```python
from build123d import *

# Parameters (mm, degrees)
STOCK_WING_STRUCTURESIZING_1_START = 350.5
STOCK_WING_STRUCTURESIZING_1_DEPTH = 3
CUT_EXTRUDE2_DEPTH                 = 278.894871602
CUT_EXTRUDE2_DEPTH_BACK            = 278.894871602
SKETCH3_R                          = 8
SKETCH3_W                          = 3
SKETCH3_H                          = 18.234468085
CUT_EXTRUDE5_DEPTH                 = 278.894871602
CUT_EXTRUDE5_DEPTH_BACK            = 278.894871602
SKETCH6_W                          = 72
SKETCH6_H                          = 36.832163157
SKETCH7_W                          = 3
SKETCH7_H                          = 29.829109924
CUT_EXTRUDE6_DEPTH                 = 3
BOSS_EXTRUDE1_DEPTH                = 3
SKETCH9_R                          = 7.192226029
SKETCH9_R_2                        = 11.636406179
SKETCH9_R_3                        = 13.307061318
SKETCH9_R_4                        = 12.161876466
SKETCH9_R_5                        = 9.990979792
SKETCH9_R_6                        = 6.753270012
CUT_EXTRUDE7_DEPTH                 = 10


# Read off the part's stored shape, not the designer's step: Stock-Wing_structureSizing-1
with BuildPart() as part:
    # Stock-Wing_structureSizing-1 outline → Stock-Wing_structureSizing-1 (new body)
    with BuildSketch(Plane.XY.offset(STOCK_WING_STRUCTURESIZING_1_START)):
        with BuildLine():
            Line((276.744987748, -9.975467242), (276.744987748, -2.791972149))
            add(Edge.make_bspline(
                [(276.744987748, -2.791972149), (265.3857023, -0.102525952), (253.985388892, 2.407220527), (231.123115134, 7.137179769), (219.66894224, 9.35664169), (202.450532833, 12.449607831), (196.704666185, 13.440005467), (185.197495984, 15.322846112), (179.436018194, 16.214183509), (167.896810084, 17.893728146), (162.119320772, 18.683464695), (150.549559093, 20.169132171), (144.757676972, 20.867539393), (133.154760401, 22.142823058), (127.340720117, 22.719276226), (115.726117513, 23.709424358), (109.921864102, 24.123286294), (92.520744809, 25.054695045), (80.935765142, 25.255529424), (63.589579679, 24.723206588), (57.812696472, 24.40777964), (49.15741104, 23.667136334), (46.27396258, 23.376378774), (40.511150261, 22.68602794), (37.631848569, 22.284778258), (31.878918329, 21.331115885), (29.005409213, 20.775520933), (24.699904445, 19.815325722), (23.265457389, 19.476044022), (20.398415094, 18.74813831), (18.963740816, 18.357002163), (16.106748162, 17.497000764), (14.692710081, 17.03099603), (11.902486035, 16.004726933), (10.526189891, 15.444736939), (8.50012674, 14.509175123), (7.830361802, 14.183402304), (6.512563898, 13.477739544), (5.865248411, 13.093583044), (4.633392785, 12.255605476), (4.045066641, 11.801499914), (3.209118512, 11.061128735), (2.938431583, 10.804207958), (2.416562808, 10.265550671), (2.165207772, 9.983507914), (1.696102707, 9.397220013), (1.477442994, 9.09171798), (1.085439515, 8.447078561), (0.915512906, 8.113897404), (0.714798114, 7.59155933), (0.657190766, 7.413573783), (0.566275814, 7.047480769), (0.533643429, 6.859526942), (0.498702003, 6.485823786), (0.495732967, 6.298500114), (0.52230969, 5.922794269), (0.553180601, 5.733657444), (0.641956646, 5.367254731), (0.699629973, 5.188174612), (0.835770495, 4.836464845), (0.914681224, 4.663114785), (1.173802922, 4.160517642), (1.376431151, 3.845824341), (1.822835658, 3.244491079), (2.068245893, 2.956719217), (2.585349641, 2.410512622), (2.856205808, 2.152934366), (3.699269455, 1.418677094), (4.302923323, 0.981675809), (5.262649419, 0.394618321), (5.591648375, 0.21018796), (6.254696782, -0.135942129), (6.589931521, -0.298692503), (7.602521133, -0.767803382), (8.28593821, -1.057311971), (9.662885491, -1.60821635), (10.357226689, -1.867357708), (12.455074514, -2.603572901), (13.873250521, -3.039868309), (16.739197416, -3.830190303), (18.188973825, -4.184254143), (22.54237297, -5.143962802), (25.459339583, -5.655261329), (31.306270814, -6.564233952), (34.235701619, -6.966574468), (40.104165427, -7.687316125), (43.043386977, -8.004069053), (51.874086741, -8.840379009), (57.778366073, -9.248032718), (66.64804678, -9.743583642), (69.60756187, -9.887823594), (75.525585547, -10.141245843), (78.484610817, -10.250077692), (84.402679828, -10.443151081), (87.361723417, -10.527595381), (93.279819329, -10.684856962), (96.238871496, -10.7578835), (111.034153794, -11.094438823), (122.870449548, -11.270610432), (140.625005024, -11.385979432), (146.54320834, -11.400264082), (158.379650661, -11.381324799), (164.297889136, -11.348805922), (176.134384089, -11.259801078), (182.052639742, -11.204415721), (193.889154401, -11.089178887), (199.807414258, -11.02819544), (217.562198328, -10.839257795), (229.398721047, -10.713290888), (253.0718283, -10.379069852), (264.908412973, -10.164021277), (276.744987748, -9.975467242)],
                knots=[0, 0, 0, 0, 0.0625, 0.0625, 0.125, 0.125, 0.15625, 0.15625, 0.1875, 0.1875, 0.21875, 0.21875, 0.25, 0.25, 0.28125, 0.28125, 0.3125, 0.3125, 0.375, 0.375, 0.40625, 0.40625, 0.421875, 0.421875, 0.4375, 0.4375, 0.453125, 0.453125, 0.4609375, 0.4609375, 0.46875, 0.46875, 0.4765625, 0.4765625, 0.484375, 0.484375, 0.48828125, 0.48828125, 0.4921875, 0.4921875, 0.49609375, 0.49609375, 0.498046875, 0.498046875, 0.5, 0.5, 0.501953125, 0.501953125, 0.50390625, 0.50390625, 0.504882813, 0.504882813, 0.505859375, 0.505859375, 0.506835938, 0.506835938, 0.5078125, 0.5078125, 0.508789063, 0.508789063, 0.509765625, 0.509765625, 0.51171875, 0.51171875, 0.513671875, 0.513671875, 0.515625, 0.515625, 0.51953125, 0.51953125, 0.521484375, 0.521484375, 0.5234375, 0.5234375, 0.52734375, 0.52734375, 0.53125, 0.53125, 0.5390625, 0.5390625, 0.546875, 0.546875, 0.5625, 0.5625, 0.578125, 0.578125, 0.59375, 0.59375, 0.625, 0.625, 0.640625, 0.640625, 0.65625, 0.65625, 0.671875, 0.671875, 0.6875, 0.6875, 0.75, 0.75, 0.78125, 0.78125, 0.8125, 0.8125, 0.84375, 0.84375, 0.875, 0.875, 0.9375, 0.9375, 1, 1, 1, 1], degree=3))
        make_face()
    extrude(amount=STOCK_WING_STRUCTURESIZING_1_DEPTH)

    # Sketch3 → Cut-Extrude2 (cut, two sides: drawn at the far end of the back side and taken through both)
    with BuildSketch(Plane.XY.offset(353.5).offset(-CUT_EXTRUDE2_DEPTH_BACK)):
        with Locations((76.810751166, 3.840845639)):
            Circle(SKETCH3_R)
        with Locations((62.810751166, 15.958079682)):
            Rectangle(SKETCH3_W, SKETCH3_H)
        with Locations((90.810751166, 15.958079682)):
            Rectangle(SKETCH3_W, SKETCH3_H)
    extrude(amount=CUT_EXTRUDE2_DEPTH + CUT_EXTRUDE2_DEPTH_BACK, mode=Mode.SUBTRACT)

    # Sketch6 → Cut-Extrude5 (cut, two sides: drawn at the far end of the back side and taken through both)
    with BuildSketch(Plane.XY.offset(353.5).offset(-CUT_EXTRUDE5_DEPTH_BACK)):
        with Locations((240.744987748, -6.383719695)):
            Rectangle(SKETCH6_W, SKETCH6_H)
    extrude(amount=CUT_EXTRUDE5_DEPTH + CUT_EXTRUDE5_DEPTH_BACK, mode=Mode.SUBTRACT)

    # Sketch7 → Cut-Extrude6 (cut)
    with BuildSketch(Plane.XY.offset(353.5)):
        with Locations((1.5, 14.914554962)):
            Rectangle(SKETCH7_W, SKETCH7_H)
    extrude(amount=-CUT_EXTRUDE6_DEPTH, mode=Mode.SUBTRACT)

    # Sketch8 → Boss-Extrude1 (add)
    with BuildSketch(Plane.XY.offset(353.5)):
        Polygon((14.079741692, 16.8), (3, 16.8), (3, 10.856999155), (0, 10.856999155), (0, 2.029447684), (3, 2.029447684), (3, 0), (5.994622402, 0), align=None)
        Polygon((204.744998472, 7.032361884), (207.744998472, 7.032361884), (207.744998472, -4.967638116), (204.744998472, -4.967638116), (202.527550965, -4.967638116), (202.527550965, 7.032361884), align=None)
    extrude(amount=-BOSS_EXTRUDE1_DEPTH)

    # Sketch9 → Cut-Extrude7 (cut)
    with BuildSketch(Plane.XY.offset(353.5)):
        with Locations((20.96232931, 6.753270012)):
            Circle(SKETCH9_R)
        with Locations((46.004691522, 7.523804234)):
            Circle(SKETCH9_R_2)
        with Locations((111.500100385, 6.753270012)):
            Circle(SKETCH9_R_3)
        with Locations((141.93620215, 5.404835124)):
            Circle(SKETCH9_R_4)
        with Locations((168.904899918, 3.478499569)):
            Circle(SKETCH9_R_5)
        with Locations((193.176727908, 1.166896903)):
            Circle(SKETCH9_R_6)
    extrude(amount=-CUT_EXTRUDE7_DEPTH, mode=Mode.SUBTRACT)


solid = part.part
```
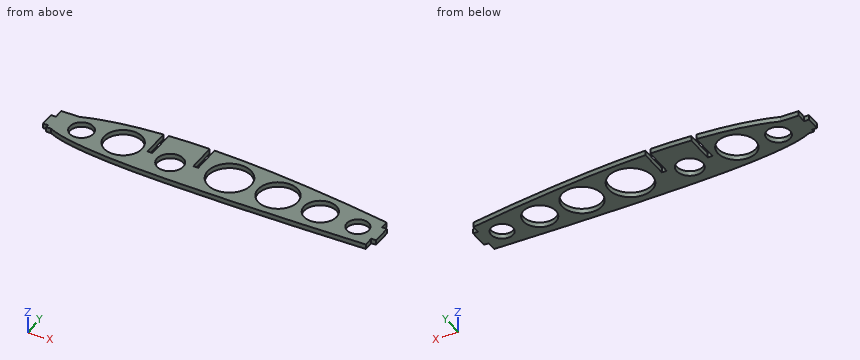
Can you work these out from the model? Positions are in its coordinate system, mm. Round coordinates to 2 decimals unless told otherwise and drop trailing zeros. Answer as a JSON object with one key per item and string values. Group by question number.
Q1. Imagine slicing it at A-A, the plane z = 352.8. Count the separate pieces of the cut face and the enclosed holes in it, then the cut area to 3 significant figures.
Q2. Please list where these lines run through material, in increasing order: L1, parallel to Y at x = 187, z = 352.65; L2, parallel to Y at x = 192.5, z = 352.9; L3, parallel to Y at x = 89, z = 351.6.
Q3. Will these pins go through, and if not, where does the flat tip stop? pin 1 (1.5 mm diameter, centred on x = 30.5, z = 351.5, fed in from -Y); pin 2 (1.6 mm diameter, centred on y = 1, z = 352.5, fed in from -X); pin 3 (0.9 mm diameter, centred on x = 2, z = 351.5, fed in from +Y).
Findings:
{
 "1": {"separate pieces": "1", "enclosed holes": "7", "area": "3,820 mm2"},
 "2": {"L1": "y = -11.16 to -1.56, 3.9 to 15.02", "L2": "y = -11.1 to -5.55, 7.89 to 14.13", "L3": "y = -10.57 to 24.99"},
 "3": {"pin 1": "stops at y = -6.54", "pin 2": "stops at x = 3", "pin 3": "stops at y = 10.86"}
}
